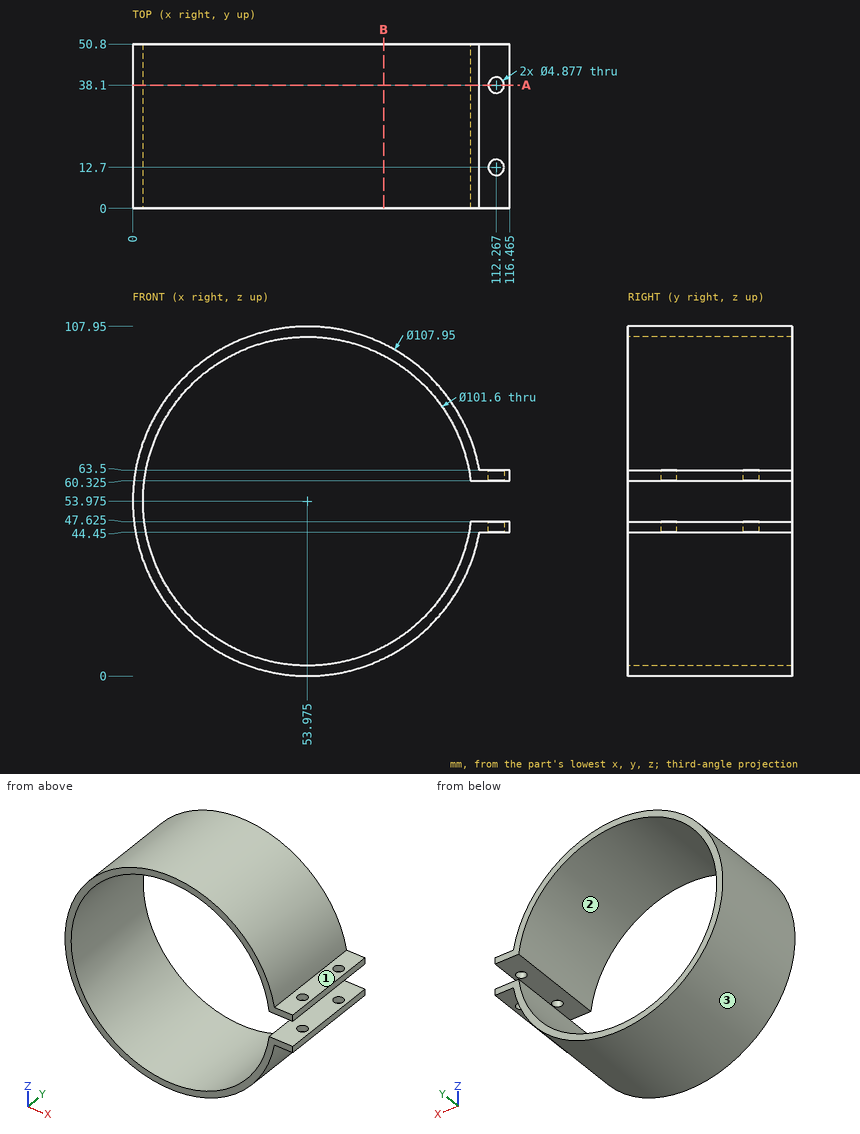
Part print with two shaded views. Sizes in mm from the minimum x, y, z corner. Give positions to 0.01 mm unless a question says otherwise; leave off trailing zeros. Order: outer loops, then holes, each group sorted by start corner. A loop starts at its lowest first (then second) coordinate and runs counter-clockwise, first axis right, second up.
1) Mould opens along Z. For the marked faces 1, 2 and 3 say: +Z half, -Z half, draft (parallel to the pull), parting line (faces both ways), or undercut.
2) Pin check, flat tips, straight feed: pin 1 (4 mm diameter, centred on x = 82, y = 40.5, fed in from +Z); pin 2 (3 mm diameter, centred on x = 113, y = 31, fed in from +Z); pin 3 (12 mm diameter, centred on x = 47.5, y = 26, fed in from +Z); pin 4 (4 mm diameter, centred on x = 112.27, y = 12.7, fed in from +Z). Stop position of each tip, or through.
3) Wall check: probe 1 along Z at (x, y) = (109.5, 31) (3 decimals); probe 2 along Z at (x, y) = (53.5, 7); probe 3 along X at (y, z) = (17.5, 10). Give the ranges that are in metal, low to high.
4) Saw through at B-B, the plane x = 77.5. Write the cut outline in (y, z), then the cut area to 3 significant figures.
5) Saw through at A-A, the plane y = 38.1. Count the separate pieces of the cut face and the enclosed holes in it, then the cut area to 3 significant figures.
Computed:
1. face 1: +Z half
1. face 2: undercut
1. face 3: parting line
2. pin 1: stops at z = 101.26
2. pin 2: stops at z = 63.5
2. pin 3: stops at z = 107.95
2. pin 4: passes through
3. probe 1: z = 44.45 to 47.625, 60.325 to 63.5
3. probe 2: z = 0 to 3.18, 104.77 to 107.95
3. probe 3: x = 22.68 to 28.54, 79.41 to 85.27
4. outline: (0, 5.4) - (50.8, 5.4) - (50.8, 8.95) - (0, 8.95) - close; (0, 99) - (50.8, 99) - (50.8, 102.55) - (0, 102.55) - close
4. area: 361 mm2
5. separate pieces: 3
5. enclosed holes: 0
5. area: 1,030 mm2
